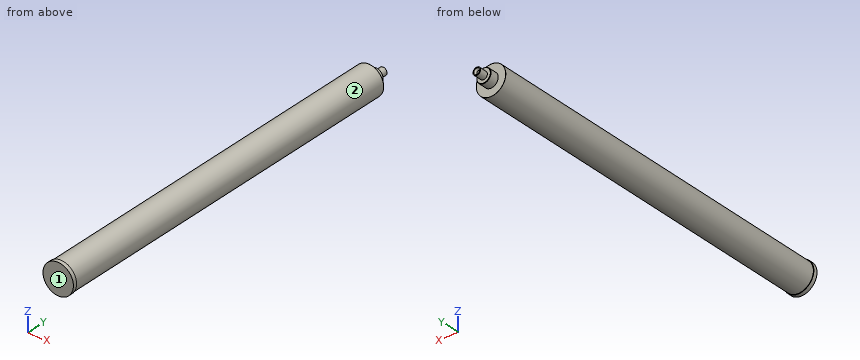
from build123d import *

# Parameters (mm, degrees)
SKETCH1_R                                           = 49.2125
BOSS_EXTRUDE1_DEPTH                                 = 1238.504
SKETCH3_R                                           = 50.8
BOSS_EXTRUDE2_DEPTH                                 = 12.7
CHAMFER1_SIZE                                       = 1.27
FILLET1_R                                           = 0.254
CSK_FOR_3_8_FLAT_HEAD_SOCKET_CAP_SCREW1_D           = 9.8044
CSK_FOR_3_8_FLAT_HEAD_SOCKET_CAP_SCREW1_DEPTH       = 25.4
CSK_FOR_3_8_FLAT_HEAD_SOCKET_CAP_SCREW1_CSINK_D     = 19.8374
CSK_FOR_3_8_FLAT_HEAD_SOCKET_CAP_SCREW1_CSINK_ANGLE = 82
CSK_FOR_3_8_FLAT_HEAD_SOCKET_CAP_SCREW1_TIP         = 2.945538927


with BuildPart() as part:
    # Sketch1 → Boss-Extrude1 (new body)
    with BuildSketch(Plane(origin=(0, 0, 0), x_dir=(1, 0, 0), z_dir=(0, 1, 0))):
        Circle(SKETCH1_R)
    extrude(amount=BOSS_EXTRUDE1_DEPTH)

    # Sketch2 → Revolve1 (revolve)
    with BuildSketch(Plane.XY):
        Polygon((0, 1238.504), (0, 1295.654), (12.7, 1295.654), (12.7, 1268.349), (23.876, 1268.349), (23.876, 1238.504), align=None)
    revolve(axis=Axis((0, 1238.504, 0), (0, 1, 0)))

    # Sketch3 → Boss-Extrude2 (add)
    with BuildSketch(Plane.XZ):
        Circle(SKETCH3_R)
    extrude(amount=BOSS_EXTRUDE2_DEPTH)

    # Chamfer1
    chamfer1_edges = [part.edges().sort_by_distance(p)[0] for p in [
        (-23.876, 1268.349, 0),
    ]]
    chamfer(chamfer1_edges, length=CHAMFER1_SIZE)

    # Fillet1
    fillet1_edges = [part.edges().sort_by_distance(p)[0] for p in [
        (-49.2125, 1238.504, 0),
    ]]
    fillet(fillet1_edges, radius=FILLET1_R)

    # CSK for 3/8 Flat Head Socket Cap Screw1
    with Locations(Plane(origin=(0, 1295.654, 0), x_dir=(1, 0, 0), z_dir=(0, 1, 0))):
        with Locations((0, 0)):
            CounterSinkHole(CSK_FOR_3_8_FLAT_HEAD_SOCKET_CAP_SCREW1_D / 2, CSK_FOR_3_8_FLAT_HEAD_SOCKET_CAP_SCREW1_CSINK_D / 2, depth=CSK_FOR_3_8_FLAT_HEAD_SOCKET_CAP_SCREW1_DEPTH, counter_sink_angle=CSK_FOR_3_8_FLAT_HEAD_SOCKET_CAP_SCREW1_CSINK_ANGLE)
            with Locations((0, 0, -(CSK_FOR_3_8_FLAT_HEAD_SOCKET_CAP_SCREW1_DEPTH + CSK_FOR_3_8_FLAT_HEAD_SOCKET_CAP_SCREW1_TIP / 2))):  # 118° drill point
                Cone(0, CSK_FOR_3_8_FLAT_HEAD_SOCKET_CAP_SCREW1_D / 2, CSK_FOR_3_8_FLAT_HEAD_SOCKET_CAP_SCREW1_TIP, mode=Mode.SUBTRACT)


solid = part.part
Source: CAD feature listing. Evaluate the final solid. Frame: model axes, mm. Face numbers are marked on the shaded views. A direction names the side the tool comes from. Give positions to 0.01 mm unless a question says otherwise; leave off trailing zeros. Write each loop counter-clockwise with the first axis right and the second up, starting at its lowest first coordinate (ties: lowest second). Pieces come first, ordered by that corner, then holes. Notation, with made-up numbers: (6.25, 84) -> (22.25, 84) arc R27 ccw to (22.25, 121) -> close; hole circle Ø7 at (-7, -25.5). An arc over 180 degrees is marked (long way). Return JSON: item names as keys, results as strings. Group by question number.
1. Material intervals for line 1 (Z direction, x = 0, y = 1276.5); line 2 (Z direction, x = -6, y = 868.5); line 3 (Y direction, x = -26, z = -17), sorted ascending. Write a range as from..to.
2. Pin query (flat end, axial travel): pin 1 Ø6 at (y, z) = (760, 22) entering from -X; pin 2 Ø3 at (y, z) = (149.5, 0.5) entering from -X; pin 3 Ø8 at (y, z) = (460.5, 14) entering from -X. Return the tip coordinate at first contact, or that it passes through.
3. Section A-A, the plane y = 94. Output: boundary loops of the cut face in (x, z) (1 decimal), then the cut area to 3 significant figures.
4. Access query for the marked faces 1 and 2. Directions: +Z, -Z, +X, -X, +Y, -Y. A direction counts if a zero-diameter tool reaches every point of the face in a straight line with its end or side. Return the directions, or none.
Determined:
{
 "1": {"line 1": "z = -12.7..-4.9, 4.9..12.7", "line 2": "z = -48.85..48.85", "line 3": "y = -12.7..1238.5"},
 "2": {"pin 1": "stops at x = -45.4", "pin 2": "stops at x = -49.21", "pin 3": "stops at x = -48.19"},
 "3": {"outline": "circle Ø98.4 at (0, 0)", "area": "7,610 mm2"},
 "4": {"face 1": "+Z, -Z, +X, -X, -Y", "face 2": "+Y"}
}
